Drawing for the job (mm, zero at the part's lowest x, y, z). A direction names the side the tool comes from. Round coordinates to 2 decimals unless told otherwise and drop trailing zeros. Write each loop counter-clockwise with the first axis right and the second up, starting at its lowest first coordinate (ties: lowest second). Pieces come first, ordered by that corner, then holes. Notation, with made-up numbers: M 56.25,8.25 L 103.25,8.25 A26 cw 103.25,22.25 Z; hole C 88,54 d7. An arc over 180 degrees is marked long. Use a Markdown table: item, result. Add a question column.
1) Wall check: probe 1 along X at (y, z) = (46, 53.5) (1 decimal); probe 2 along Y at (x, z) = (92, 58.5); probe 3 along X at (y, z) = (29, 36.5) (1 decimal). Give the ranges that are in metal, low to high.
2) Slice it at B-B on x = 66.5. Write the cut outline in (y, z).
3) Slice it at D-D on z = 15. Write the cut outline in (x, y), plus the area to 3 significant figures.
4) Slice it at C-C on x = 104.5. Write the cut outline in (y, z).
5) Which spindle directions (+Z, -Z, +X, -X, +Y, -Y) get a long thin tool onto all of the face, cutting with end or side? Do the marked faces 1 and 2. Say none if no direction does.
6) Slice it at A-A on y = 29. Write the cut outline in (x, z).
7) Drop a flat-ended pin along its axis: P1, Ø6, axis at x = 86.5, z = 10, coming from the -Y side. Give the stop position or say it passes through.
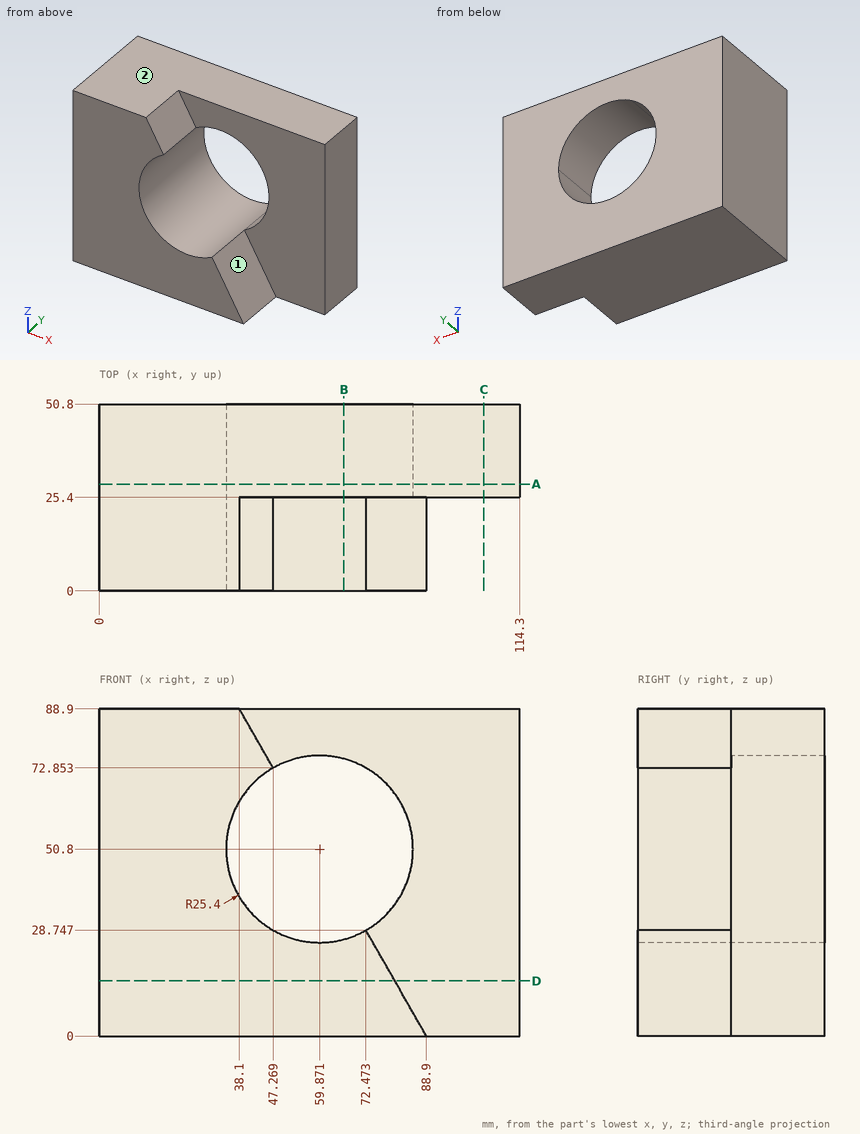
Entries:
| question | item | result |
|---|---|---|
| 1 | probe 1 | x = 0 to 34.6, 85.1 to 114.3 |
| 1 | probe 2 | y = 25.4 to 50.8 |
| 1 | probe 3 | x = 0 to 38.9, 80.9 to 114.3 |
| 2 | outline | M 0,0 L 50.8,0 L 50.8,26.28 L 0,26.28 Z; M 25.4,75.32 L 50.8,75.32 L 50.8,88.9 L 25.4,88.9 Z |
| 3 | outline | M 0,0 L 80.33,0 L 80.33,25.4 L 114.3,25.4 L 114.3,50.8 L 0,50.8 Z |
| 3 | area | 4,940 mm^2 |
| 4 | outline | M 25.4,0 L 50.8,0 L 50.8,88.9 L 25.4,88.9 Z |
| 5 | face 1 | +Z, +X, -Y |
| 5 | face 2 | +Z, +X, -X, +Y, -Y |
| 6 | outline | M 0,0 L 114.3,0 L 114.3,88.9 L 0,88.9 Z; hole M 72.47,28.75 A25.4 ccw 85.27,50.8 A25.4 ccw long Z |
| 7 | P1 | stops at y = 0 |
